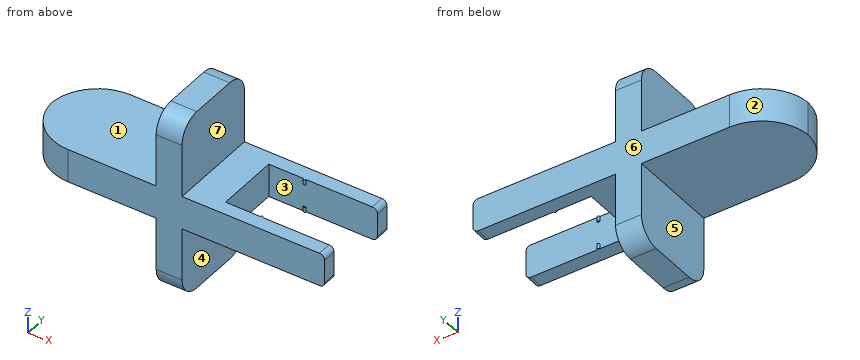
from build123d import *

# Parameters (mm, degrees)
BOSS_EXTRUDE1_DEPTH = 4.92
CUT_EXTRUDE1_REACH  = 27.419
CUT_EXTRUDE2_REACH  = 24.607
SKETCH3_W           = 3.42
SKETCH3_H           = 9.3
BOSS_EXTRUDE2_DEPTH = 3.81
SKETCH5_W           = 4.92
SKETCH5_H           = 13.42
BOSS_EXTRUDE3_DEPTH = 20
FILLET1_R           = 7


with BuildPart() as part:
    # Sketch1 → Boss-Extrude1 (new body)
    with BuildSketch(Plane.XY):
        with BuildLine():
            Line((0, -6.71), (0, 6.71))
            Line((0, 6.71), (21.02, 6.71))
            Line((21.02, 6.71), (21.02, 4.65))
            Line((21.02, 4.65), (10.52, 4.65))
            ThreePointArc((10.52, 4.65), (10.32, 4.45), (10.12, 4.65))
            Line((10.12, 4.65), (5, 4.65))
            Line((5, 4.65), (5, -4.65))
            Line((5, -4.65), (10.12, -4.65))
            ThreePointArc((10.12, -4.65), (10.32, -4.45), (10.52, -4.65))
            Line((10.52, -4.65), (21.02, -4.65))
            Line((21.02, -4.65), (21.02, -6.71))
            Line((21.02, -6.71), (0, -6.71))
        make_face()
    extrude(amount=BOSS_EXTRUDE1_DEPTH)

    # Cut-Extrude1: up to this face of the body (flat: up to its plane)
    cut_extrude1_end = Plane(part.part.faces().sort_by_distance((10.51, -6.71, 2.46))[0])
    # Sketch2 → Cut-Extrude1 (cut, up to the picked face)
    with BuildSketch(Plane(origin=(0, 6.71, 0), x_dir=(1, 0, 0), z_dir=(0, 1, 0)), mode=Mode.PRIVATE) as cut_extrude1_sk1:
        with BuildLine():
            Line((18.617685134, -4.92), (20.27, -4.92))
            ThreePointArc((20.27, -4.92), (20.800330086, -4.700330086), (21.02, -4.17))
            Line((21.02, -4.17), (21.02, -0.75))
            ThreePointArc((21.02, -0.75), (20.800330086, -0.219669914), (20.27, 0))
            Line((20.27, 0), (18.617685134, 0))
            Line((18.617685134, 0), (18.617685134, 2.663079407))
            Line((18.617685134, 2.663079407), (23.784387399, 2.663079407))
            Line((23.784387399, 2.663079407), (23.784387399, -9.532215778))
            Line((23.784387399, -9.532215778), (18.617685134, -9.532215778))
            Line((18.617685134, -9.532215778), (18.617685134, -4.92))
        make_face()
    cut_extrude1_tool1 = split(extrude(cut_extrude1_sk1.sketch, amount=-CUT_EXTRUDE1_REACH, mode=Mode.PRIVATE), bisect_by=cut_extrude1_end, keep=Keep.BOTH, mode=Mode.PRIVATE)
    add(cut_extrude1_tool1.solids().sort_by(Axis((21.51704, 6.71, 3.653957), (0, -1, 0)))[0], mode=Mode.SUBTRACT)

    # Cut-Extrude2: up to this face of the body (flat: up to its plane)
    cut_extrude2_end = Plane(part.part.faces().sort_by_distance((5, 0, 2.46))[0])
    # Sketch3 → Cut-Extrude2 (cut, up to the picked face)
    with BuildSketch(Plane(origin=(21.02, 0, 0), x_dir=(0, 0, -1), z_dir=(1, 0, 0)), mode=Mode.PRIVATE) as cut_extrude2_sk1:
        with Locations((-2.46, 0)):
            Rectangle(SKETCH3_W, SKETCH3_H)
    cut_extrude2_tool1 = split(extrude(cut_extrude2_sk1.sketch, amount=-CUT_EXTRUDE2_REACH, mode=Mode.PRIVATE), bisect_by=cut_extrude2_end, keep=Keep.BOTH, mode=Mode.PRIVATE)
    add(cut_extrude2_tool1.solids().sort_by(Axis((21.02, 0, 2.46), (-1, 0, 0)))[0], mode=Mode.SUBTRACT)

    # Sketch4 → Boss-Extrude2 (add)
    with BuildSketch(Plane.ZY):
        with BuildLine():
            Line((12.705, -6.71), (-7.785, -6.71))
            ThreePointArc((-7.785, -6.71), (-10.03006403, -5.78006403), (-10.96, -3.535))
            Line((-10.96, -3.535), (-10.96, 3.535))
            ThreePointArc((-10.96, 3.535), (-10.03006403, 5.78006403), (-7.785, 6.71))
            Line((-7.785, 6.71), (12.705, 6.71))
            ThreePointArc((12.705, 6.71), (14.95006403, 5.78006403), (15.88, 3.535))
            Line((15.88, 3.535), (15.88, -3.535))
            ThreePointArc((15.88, -3.535), (14.95006403, -5.78006403), (12.705, -6.71))
        make_face()
    extrude(amount=BOSS_EXTRUDE2_DEPTH)

    # Sketch5 → Boss-Extrude3 (add)
    with BuildSketch(Plane.ZY.offset(3.81)):
        with Locations((2.46, 0)):
            Rectangle(SKETCH5_W, SKETCH5_H)
    extrude(amount=BOSS_EXTRUDE3_DEPTH)

    # Fillet1
    # the kernel refuses this fillet: 7 mm, written as the material it takes off along each edge
    with BuildSketch(Plane(origin=(-23.81, -6.71, 22.42), x_dir=(1, 0, 0), z_dir=(0, 0, -1)), Plane(origin=(-23.81, 6.71, -17.5), x_dir=(1, 0, 0), z_dir=(0, 0, 1))) as fillet1_piece_1:
        with BuildLine():
            CenterArc((FILLET1_R, -FILLET1_R), FILLET1_R, 90, 90)
            Line((0, -FILLET1_R), (0, 0))
            Line((0, 0), (FILLET1_R, 0))
        make_face()
    extrude(amount=39.92, mode=Mode.SUBTRACT)


solid = part.part
Read the model definition and answer for the solid it produces. Units are mm, in the model's axes. Face numbers are marked on the shaded views. A direction names the side the tool comes from. Give positions to 0.01 mm unless a question says otherwise; leave off trailing zeros. Write each loop counter-clockwise with the first axis right and the second up, starting at its lowest first coordinate (ties: lowest second). Pieces come first, ordered by that corner, then holes. Notation, with made-up numbers: (19.25, 43.5) -> (75.25, 43.5) arc R36 ccw to (75.25, 79.5) -> close; hole circle Ø2 at (-20, 46). An arc over 180 degrees is marked (long way). Answer as a JSON object with one key per item and string values. Group by question number.
1) Find section C-C (x = -9.5). Write down the section's boundary in (y, z), and give its area (3 significant figures).
2) Find section D-D (y = -2.5). Write down the section's boundary in (x, z).
3) Find section A-A (z = 3.5). Write down the section's boundary in (x, y), and give its area (3 significant figures).
4) A tool of negligible diameter and unlimited length cuts with its end or side. For the marked faces 4, 5, 6 and 7, from which of +Z, -Z, +X, -X, +Y, -Y can it reach the whole face along a straight path? Write none if from no direction.
5) Find section B-B (y = -0.5). Write down the section's boundary in (x, z).
6) The mould has two halves that part along Y. Classify the marked faces 1, 2 and 3: +Y half, -Y half, draft (parallel to the pull), parting line (faces both ways), or undercut.
7) Each of these flat-tipped pins is pushed along its axis until it touches: P1, Ø4, axis at y = 2, z = -3.5, coming from the +X side; P2, Ø4, axis at y = 5, z = 2.5, coming from the -X side; P3, Ø5, axis at x = 0.5, y = -4.5, coming from the +Z side; P4, Ø3, axis at x = -17.5, y = -3, coming from the -Z side. Where does it stop, or does it pass through?
8) Consider L1, parallel to Y at x = 8.5, z = 3.75; L2, parallel to X at y = 0, z = -7.5; L3, parallel to Z at x = -6, y = 2.5. Determine where each line is inside the solid, lowest interval first. Write a range as from..to.
Values follow:
{
 "1": {"outline": "(-6.71, 0) -> (6.71, 0) -> (6.71, 4.92) -> (-6.71, 4.92) -> close", "area": "66.0 mm2"},
 "2": {"outline": "(-23.23, 0) -> (-3.81, 0) -> (-3.81, -10.96) -> (0, -10.96) -> (0, 0) -> (5, 0) -> (5, 4.92) -> (0, 4.92) -> (0, 15.88) -> (-3.81, 15.88) -> (-3.81, 4.92) -> (-23.23, 4.92) -> close"},
 "3": {"outline": "(-23.8, 0) arc R7 ccw to (-16.81, -6.71) -> (21.02, -6.71) -> (21.02, -4.65) -> (5, -4.65) -> (5, 4.65) -> (21.02, 4.65) -> (21.02, 6.71) -> (-16.81, 6.71) arc R7 ccw to start", "area": "432 mm2"},
 "4": {"face 4": "-Z, +X, +Y, -Y", "face 5": "-Z, -X, +Y, -Y", "face 6": "+Z, -Z, +X, -X, +Y", "face 7": "+Z, +X, +Y, -Y"},
 "5": {"outline": "(-23.77, 0) -> (-3.81, 0) -> (-3.81, -10.96) -> (0, -10.96) -> (0, 0) -> (5, 0) -> (5, 4.92) -> (0, 4.92) -> (0, 15.88) -> (-3.81, 15.88) -> (-3.81, 4.92) -> (-23.77, 4.92) -> close"},
 "6": {"face 1": "draft", "face 2": "+Y half", "face 3": "undercut"},
 "7": {"P1": "stops at x = 0", "P2": "stops at x = -22.99", "P3": "stops at z = 15.88", "P4": "stops at z = 0"},
 "8": {"L1": "y = -6.71..-4.65, 4.65..6.71", "L2": "x = -3.81..0", "L3": "z = 0..4.92"}
}
